```python
from build123d import *

# Parameters (mm, degrees)
F0_W      = 74
F0_H      = 30
F1_DEPTH  = 21
F2_SIZE2  = 34
F2_SIZE   = 10
F3_W      = 30
F3_H      = 30
F4_DEPTH  = 20
F5_R      = 10
F6_DEPTH  = 50.001
F7_R      = 6
F8_DEPTH  = 35.001
F10_W     = 12
F10_H     = 20
F11_DEPTH = 30.0010001
F9_R      = 15
F12_DEPTH = 74.001


with BuildPart() as f1:
    # F0 (on Right) → F1 (new body, symmetric)
    with BuildSketch(Plane.YZ):
        Rectangle(F0_W, F0_H)
    extrude(amount=F1_DEPTH, both=True)

    # F2
    f2_edges = [f1.edges().sort_by_distance(p)[0] for p in [
        (0, -37, 15),
    ]]
    f2_side = f1.faces().sort_by_distance((0, -37, 0))[0]
    chamfer(f2_edges, length=F2_SIZE, length2=F2_SIZE2, reference=f2_side)

    # F3 (on face) → F4 (join)
    with BuildSketch(Plane.XY.offset(15)):
        with Locations((0, 17)):
            Rectangle(F3_W, F3_H)
    extrude(amount=F4_DEPTH)

    # F5 (on face) → F6 (cut, through all)
    with BuildSketch(Plane.XY.offset(35)):
        with Locations((0, 17)):
            Circle(F5_R)
    extrude(amount=-F6_DEPTH, mode=Mode.SUBTRACT)

    # F7 (on face) → F8 (cut, through all)
    with BuildSketch(Plane.XZ.offset(-2)):
        with Locations((0, 25)):
            Circle(F7_R)
    extrude(amount=-F8_DEPTH, mode=Mode.SUBTRACT)

    # F10 (on face) → F11 (cut, through all)
    with BuildSketch(Plane.XY.offset(15)):
        with Locations((0, -20)):
            Rectangle(F10_W, F10_H)
    extrude(amount=-F11_DEPTH, mode=Mode.SUBTRACT)

    # F9 (on face) → F12 (cut, through all)
    with BuildSketch(Plane.XZ.offset(37)):
        with Locations((0, -15)):
            Circle(F9_R)
    extrude(amount=-F12_DEPTH, mode=Mode.SUBTRACT)


solid = f1.part
```
Build history of the part. All positions in model axes, mm. A direction names the side the tool comes from. Round coordinates to 2 decimals unless told otherwise and drop trailing zeros. Write each loop counter-clockwise with the first axis right and the second up, starting at its lowest first coordinate (ties: lowest second). Pieces come first, ordered by that corner, then holes. Notation, with made-up numbers: (67.25, 31) - (93.25, 31) arc R31 ccw to (93.25, 60) - close; hole circle Ø5 at (-20, -19). An arc over 180 degrees is marked (long way). Write each question's results on one line, items separated by ' | '. Start each with the question number.
Item 1: Saw through at A-A (y = -11.5). Write the cut outline in (x, z).
Item 2: Saw through at B-B (z = 25). Write the cut outline in (x, y), and give its area (3 significant figures).
Item 3: Saw through at D-D (y = 30). Write the cut outline in (x, z).
Item 4: Wall check: L1, parallel to Z at x = 0, y = 30; L2, parallel to X at y = 17, z = 4.5; L3, parallel to X at y = 27, z = 25. Give the ranges that are in metal, low to high. Write a range as [from, to].
Item 5: Drop flat-ended pins along their axis: P1, Ø22, axis at x = 4, z = 27, coming from the -Y side; P2, Ø7, axis at x = 0, z = 25, coming from the +Y side; P3, Ø16, axis at y = 20.5, z = 25.5, coming from the -X side; P4, Ø2, axis at x = 13.5, y = -0.5, coming from the +Z side. Give the stop position or say it passes through.
Item 6: Which spindle directions (+Z, -Z, +X, -X, +Y, -Y) get a long thin tool onto all of the face, cutting with end or side? Do faces 5 (the face through (5.723, 29.229, 26.802)), 6 (the face through (0, 32, 32)), 7 (the face through (6, -20, 4)), 8 (the face through (15, 17, 25)). Say none if no direction does.
Item 7: Mould opens along Y. For faces 1 (the face through (-7.37, 23.76, 15.86)), 2 (the face through (-18, -1, -15)), 3 (the face through (0, 37, 3)), 4 (the face through (-6, -20, 4)) say: pulls with the +Y half, pulls with the -Y half, needs draft (parallel to the pull), parting line crosses it, or undercut.
Item 8: Saw through at C-C (z = 6). Write the cut outline in (x, y), and give its area (3 significant figures).
Results are:
1) outline: (-21, -15) - (-15, -15) arc R15 cw to (-6, -1.25) - (-6, 12.5) - (-21, 12.5) - close; (6, -1.25) arc R15 cw to (15, -15) - (21, -15) - (21, 12.5) - (6, 12.5) - close
2) outline: (-15, 2) - (-6, 2) - (-6, 9) arc R10 cw to (-6, 25) - (-6, 32) - (-15, 32) - close; (6, 2) - (15, 2) - (15, 32) - (6, 32) - (6, 25) arc R10 cw to (6, 9) - close | area: 451 mm²
3) outline: (-21, -15) - (-15, -15) arc R15 cw to (15, -15) - (21, -15) - (21, 15) - (15, 15) - (15, 35) - (-15, 35) - (-15, 15) - (-21, 15) - close; hole circle Ø12 at (0, 25)
4) L1: z = [0, 19], [31, 35] | L2: x = [-21, -10], [10, 21] | L3: x = [-15, -6], [6, 15]
5) P1: stops at y = 2 | P2: passes through | P3: stops at x = -15 | P4: stops at z = 15
6) face 5: +Y, -Y | face 6: +Z, +X, -X, +Y | face 7: +Z, -Z | face 8: +Z, +X, +Y, -Y
7) face 1: undercut | face 2: needs draft | face 3: pulls with the +Y half | face 4: undercut
8) outline: (-21, -33.6) - (21, -33.6) - (21, 37) - (-21, 37) - close; hole circle Ø20 at (0, 17); hole (-6, -30) - (6, -30) - (6, -10) - (-6, -10) - close | area: 2,410 mm²
